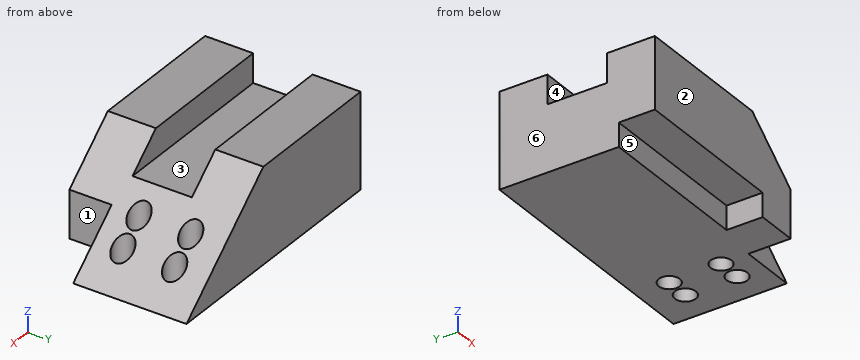
```python
from build123d import *

# Parameters (mm, degrees)
F1_DEPTH  = 76.2
F3_W      = 58.20692
F3_H      = 57.454397
F4_DEPTH  = 215.138
F6_DEPTH  = 154.686
F7_W      = 56.875151
F7_H      = 62.153444
F8_DEPTH  = 41.402
F9_W      = 44.515941
F9_H      = 35.404432
F10_DEPTH = 154.94
F11_R     = 10.245483
F12_DEPTH = 93.251692


with BuildPart() as f1:
    # F0 (on Front) → F1 (new body, symmetric)
    with BuildSketch(Plane.XZ):
        Polygon((69.90508, 46.625346), (-69.90508, 46.625346), (-69.90508, -46.625346), (69.90508, -46.625346), (180.455416, -46.625346), align=None)
    extrude(amount=F1_DEPTH, both=True)

    # F3 (on face) → F4 (cut)
    with BuildSketch(Plane(origin=(-69.90508, 0, 0), x_dir=(0, -1, 0), z_dir=(-1, 0, 0))):
        with Locations((0, 46.984415)):
            Rectangle(F3_W, F3_H)
    extrude(amount=-F4_DEPTH, mode=Mode.SUBTRACT)

    # F5 (on face) → F6 (cut)
    with BuildSketch(Plane.XZ.offset(76.2)):
        Polygon((185.93514, 8.272756), (115.37275, 8.272756), (180.455416, -46.625346), (115.37275, -46.625346), (115.37275, -61.852183), (185.93514, -61.852183), align=None)
    extrude(amount=-F6_DEPTH, mode=Mode.SUBTRACT)

    # F7 (on face) → F8 (cut)
    with BuildSketch(Plane.XZ.offset(76.2)):
        with Locations((153.617823, -31.076722)):
            Rectangle(F7_W, F7_H)
    extrude(amount=-F8_DEPTH, mode=Mode.SUBTRACT)

    # F9 (on face) → F10 (cut)
    with BuildSketch(Plane(origin=(-69.90508, 0, 0), x_dir=(0, -1, 0), z_dir=(-1, 0, 0))):
        with Locations((63.042035, -41.065147)):
            Rectangle(F9_W, F9_H)
    extrude(amount=-F10_DEPTH, mode=Mode.SUBTRACT)

    # F11 (on face) → F12 (cut, through all)
    with BuildSketch(Plane(origin=(0, 0, -46.625346), x_dir=(1, 0, 0), z_dir=(0, 0, -1))):
        with Locations((148.977362, 7.559244)):
            Circle(F11_R)
        with Locations((148.977362, -43.140469)):
            Circle(F11_R)
        with Locations((125.823924, 7.559244)):
            Circle(F11_R)
        with Locations((125.823924, -43.140469)):
            Circle(F11_R)
    extrude(amount=-F12_DEPTH, mode=Mode.SUBTRACT)


solid = f1.part
```
Read the model definition and answer for the solid it produces. Units are mm, in the model's axes. Face numbers are marked on the shaded views. A direction names the side the tool comes from. Give positions to 0.01 mm unless a question says otherwise; leave off trailing zeros. Order: outer loops, then holes, each group sorted by start corner. A loop starts at its lowest first (then second) coordinate and runs counter-clockwise, first axis right, second up. Notation, with made-up numbers: (53, -17.75) -> (93, -17.75) arc R29 cw to (93, 8.25) -> close; hole circle Ø11 at (-10.5, 11). An arc over 180 degrees is marked (long way). One line per item, written item: value. Start each with the question number.
(1) The part is cut by section D-D (x = 53.5). Determine the outline of the cut face in (y, z).
(2) A tool of negligible diameter and unlimited length cuts with its end or side. For the marked faces 4, 5 and 6, from which of +Z, -Z, +X, -X, +Y, -Y can it reach the whole face along a straight path? Write none if from no direction.
(3) The part is cut by section A-A (y = -14). Determine the outline of the cut face in (x, z).
(4) Flat-ended cylindrical pins translate along their axes: P1, Ø1.5, axis at x = 20.5, y = -11, coming from the +Z side; P2, Ø12.5, axis at y = -60.5, z = -27, coming from the +X side; P3, Ø7, axis at x = 12, z = -38, coming from the -Y side. Find the tip coordinate at first contact, or state that the pin passes through.
(5) Straight lines are drawn through the part: L1, parallel to Y at x = -57, z = 22.5; L2, parallel to X at y = 43.5, z = -14.5; L3, parallel to Y at x = 118, z = 2. For each, find the intervals that lie inside material, in ascending order.
(6) For a pull along Y with two mould halves and no side action, classify the marked faces 1, 2 and 3 as released by +Y, released by -Y, zero draft, split by the parting line, or undercut.
(7) The part is cut by section C-C (x = 120.5). Determine the outline of the cut face in (y, z).
(8) The part is cut by section B-B (z = 35.5). Determine the outline of the cut face in (x, y).
Taken from the geometry:
1. outline: (-76.2, -23.36) -> (-40.78, -23.36) -> (-40.78, -46.63) -> (76.2, -46.63) -> (76.2, 46.63) -> (29.1, 46.63) -> (29.1, 18.26) -> (-29.1, 18.26) -> (-29.1, 46.63) -> (-76.2, 46.63) -> close
2. face 4: +Z, +X, -X
2. face 5: -Z, -X, -Y
2. face 6: +Z, -Z, -X, +Y, -Y
3. outline: (-69.91, -46.63) -> (117.86, -46.63) -> (117.86, 6.18) -> (103.54, 18.26) -> (-69.91, 18.26) -> close; (133.79, -46.63) -> (141.01, -46.63) -> (141.01, -13.35) -> (133.79, -7.26) -> close; (156.95, -46.63) -> (180.46, -46.63) -> (156.95, -26.79) -> close
4. P1: z = 18.26
4. P2: x = 125.18
4. P3: y = -40.78
5. L1: -76.2 to -29.1, 29.1 to 76.2
5. L2: -69.91 to 115.58, 136.06 to 138.74
5. L3: -76.2 to -14.17, -0.94 to 36.53, 49.76 to 76.2
6. face 1: zero draft
6. face 2: released by -Y
6. face 3: undercut
7. outline: (-76.2, -46.63) -> (-16.31, -46.63) -> (-16.31, 3.95) -> (-76.2, 3.95) -> close; (1.19, -46.63) -> (34.39, -46.63) -> (34.39, 3.95) -> (1.19, 3.95) -> close; (51.89, -46.63) -> (76.2, -46.63) -> (76.2, 3.95) -> (51.89, 3.95) -> close
8. outline: (-69.91, -76.2) -> (83.09, -76.2) -> (83.09, -29.1) -> (-69.91, -29.1) -> close; (-69.91, 29.1) -> (83.09, 29.1) -> (83.09, 76.2) -> (-69.91, 76.2) -> close
